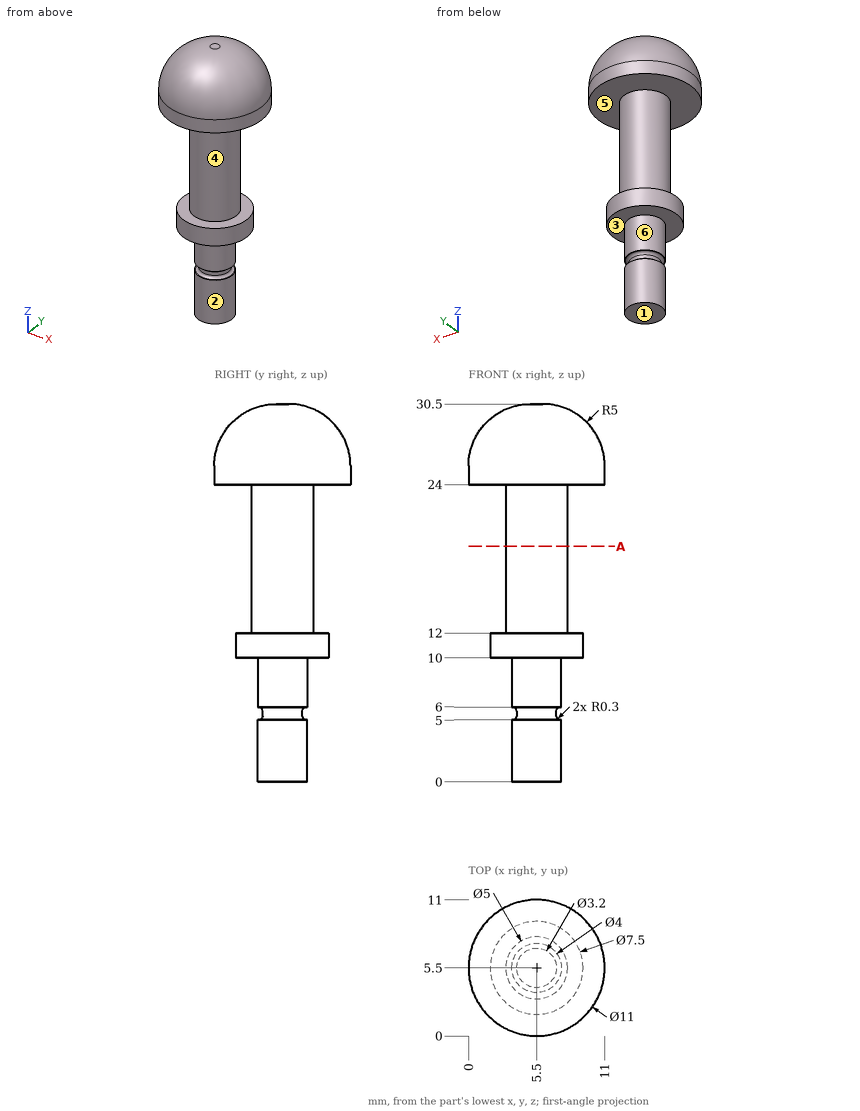
Input: dimensioned drawing with shaded views. Units: mm. Origin: part minimum x, y, z. A direction names the side the tool comes from. Give positions to 0.01 mm unless a question says otherwise; leave off trailing zeros. Write each loop counter-clockwise with the first axis right and the second up, starting at its lowest first coordinate (ties: lowest second). Pieces come first, ordered by that corner, then holes.
Q1. Material intervals for probe 1 along X at (y, z) = (7, 12.5); probe 2 along Z at (x, y) = (7.25, 7.5), sorted ascending.
Q2. Set-up query: the marked faces 1 and 2. Return all of +Z, -Z, +X, -X, +Y, -Y with unobstructed straight access to the full face (end or side cutting, diameter ignored); none if empty.
Q3. First-contact query: P1, Ø1.5, axis at y = 3.5, z = 8.5, coming from the +X side; P2, Ø6, axis at x = 7, z = 4, coming from the +Y side; P3, Ø3, axis at y = 2, z = 24, coming from the +X side. Flat tips, straight axial feed; report the tip coordinate or a pass-through.
Q4. Section A-A, the plane z = 19. Output: boundary loops of the cut face in (x, y), plus the area to 3 significant figures.
Q5. Pull-direction query (Z, two-part tool) for the marked faces 3, 4, 5 and 6; classes: pulls with the +Z half, pulls with the -Z half, needs draft (parallel to the pull), parting line crosses it, or undercut.
Filled in:
1. probe 1: x = 3.5 to 7.5
1. probe 2: z = 10 to 12, 24 to 30.01
2. face 1: -Z, +X, -X, +Y, -Y
2. face 2: -Z
3. P1: stops at x = 7.06
3. P2: stops at y = 7.5
3. P3: stops at x = 10.62
4. outline: circle Ø5 at (5.5, 5.5)
4. area: 19.6 mm2
5. face 3: pulls with the -Z half
5. face 4: undercut
5. face 5: undercut
5. face 6: needs draft
